Verification items for the finished model (mm, model axes). Face numbers are marked on the shaded views. A direction names the side the tool comes from. Round coordinates to 2 decimals unless told otherwise and drop trailing zeros. Write each loop counter-clockwise with the first axis right and the second up, starting at its lowest first coordinate (ties: lowest second). Pieces come first, ordered by that corner, then holes. Notation, with made-up numbers: (-34.5, 86) - (-21.5, 86) arc R19 ccw to (-21.5, 116) - close; hole circle Ø4 at (-23, -38.5). An arc over 180 degrees is marked (long way). Answer as a JSON object with one key per item and string values.
```python
from build123d import *

# Parameters (mm, degrees)
DODANIE_WYCI_GNI_CIE1_DEPTH = 16
SKORUPA1_T                  = -1.5
WYTNIJ_WYCI_GNI_CIE2_REACH  = 21
SZKIC12_R                   = 2.5
WYTNIJ_WYCI_GNI_CIE3_REACH  = 21
SZKIC13_R                   = 4


with BuildPart() as part:
    # Szkic1 → Dodanie-wyciągnięcie1 (new body)
    with BuildSketch(Plane.XY):
        with BuildLine():
            Line((0.5, 0), (18.5, 0))
            ThreePointArc((18.5, 0), (18.853553391, 0.146446609), (19, 0.5))
            Line((19, 0.5), (19, 20.5))
            ThreePointArc((19, 20.5), (18.853553391, 20.853553391), (18.5, 21))
            Line((18.5, 21), (0.5, 21))
            ThreePointArc((0.5, 21), (0.146446609, 20.853553391), (0, 20.5))
            Line((0, 20.5), (0, 0.5))
            ThreePointArc((0, 0.5), (0.146446609, 0.146446609), (0.5, 0))
        make_face()
    extrude(amount=DODANIE_WYCI_GNI_CIE1_DEPTH)

    # Skorupa1
    skorupa1_openings = [part.faces().sort_by_distance(p)[0] for p in [
        (9.5, 10.5, 16),
        (9.5, 10.5, 0),
    ]]
    offset(amount=SKORUPA1_T, openings=skorupa1_openings, kind=Kind.INTERSECTION)

    # Szkic12 → Wytnij-wyciągnięcie2 (cut, up to next)
    with BuildSketch(Plane.ZY, mode=Mode.PRIVATE) as wytnij_wyci_gni_cie2_sk1:
        with Locations((8, 10.5)):
            Circle(SZKIC12_R)
    wytnij_wyci_gni_cie2_tool1 = extrude(wytnij_wyci_gni_cie2_sk1.sketch, amount=-WYTNIJ_WYCI_GNI_CIE2_REACH, mode=Mode.PRIVATE) & part.part
    add(wytnij_wyci_gni_cie2_tool1.solids().sort_by_distance((0, 10.5, 8))[0], mode=Mode.SUBTRACT)

    # Szkic13 → Wytnij-wyciągnięcie3 (cut, up to next)
    with BuildSketch(Plane(origin=(19, 0, 0), x_dir=(0, 0, -1), z_dir=(1, 0, 0)), mode=Mode.PRIVATE) as wytnij_wyci_gni_cie3_sk1:
        with Locations((-8, 10.5)):
            Circle(SZKIC13_R)
    wytnij_wyci_gni_cie3_tool1 = extrude(wytnij_wyci_gni_cie3_sk1.sketch, amount=-WYTNIJ_WYCI_GNI_CIE3_REACH, mode=Mode.PRIVATE) & part.part
    add(wytnij_wyci_gni_cie3_tool1.solids().sort_by_distance((19, 10.5, 8))[0], mode=Mode.SUBTRACT)


solid = part.part
```
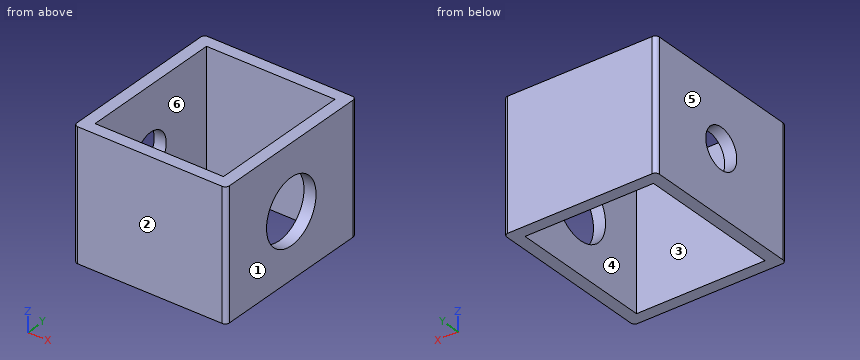
1. Material ranges on probe 1 along Y at (x, z) = (10.5, 9); probe 2 along X at (y, z) = (14, 3.25); probe 3 along Y at (x, z) = (17.8, 8), recorded low to high. Write a range as from..to.
Completed:
{"probe 1": "y = 0..1.5, 19.5..21", "probe 2": "x = 0..1.5, 17.5..19", "probe 3": "y = 0..6.5, 14.5..21"}
2. Cross-section at D-D (x = 15.75). Record the boundary of the cut face in (y, z).
Completed:
{"outline": "(0, 0) - (1.5, 0) - (1.5, 16) - (0, 16) - close; (19.5, 0) - (21, 0) - (21, 16) - (19.5, 16) - close"}
3. Access from +Z, -Z, +X, -X, +Y, -Y to the whole of each face (thin tool, end or side, straight path). Record for the marked faces 5 and 6.
Completed:
{"face 5": "+Z, -Z, -X, +Y, -Y", "face 6": "+Z, -Z"}
4. Cross-section at B-B (z = 8). Record the boundary of the cut face in (x, y), plus the area to 3 significant figures.
Completed:
{"outline": "(0, 0.5) arc R0.5 ccw to (0.5, 0) - (18.5, 0) arc R0.5 ccw to (19, 0.5) - (19, 6.5) - (17.5, 6.5) - (17.5, 1.5) - (1.5, 1.5) - (1.5, 8) - (0, 8) - close; (0, 13) - (1.5, 13) - (1.5, 19.5) - (17.5, 19.5) - (17.5, 14.5) - (19, 14.5) - (19, 20.5) arc R0.5 ccw to (18.5, 21) - (0.5, 21) arc R0.5 ccw to (0, 20.5) - close", "area": "91.3 mm^2"}
5. Mould release check, pull along Y, two halves, no side actions. Record for the marked faces 1, 2, 3 and 4: released by +Y, released by -Y, zero draft, split by the parting line, or undercut.
Completed:
{"face 1": "zero draft", "face 2": "released by -Y", "face 3": "undercut", "face 4": "undercut"}
6. Cross-section at A-A (y = 2.5). Record the boundary of the cut face in (x, z), plus the area to 3 significant figures.
Completed:
{"outline": "(0, 0) - (1.5, 0) - (1.5, 16) - (0, 16) - close; (17.5, 0) - (19, 0) - (19, 16) - (17.5, 16) - close", "area": "48.0 mm^2"}
7. Cross-section at C-C (y = 10.5). Record the boundary of the cut face in (x, z).
Completed:
{"outline": "(0, 0) - (1.5, 0) - (1.5, 5.5) - (0, 5.5) - close; (0, 10.5) - (1.5, 10.5) - (1.5, 16) - (0, 16) - close; (17.5, 0) - (19, 0) - (19, 4) - (17.5, 4) - close; (17.5, 12) - (19, 12) - (19, 16) - (17.5, 16) - close"}
